Geometry: see drawing. Coordinates: mm, zero at the bounding-box minimum. Round coordinates to 2 decimals unless told otherwise and drop trailing zeros. Loops run counter-clockwise (first coordinate to the right, second up) from the corner with the lowest first, then second, coordinate; pieces in that order, holes last.
(1) Line query: line 1 (X direction, y = 1.55, z = 105); line 2 (Z direction, x = 5, y = 2.95); line 3 (Z direction, x = 5.5, y = 1.7). Output: solid intervals per line, ascending.
(2) Cut plane A-A, the plane z = 105. Output: boundary loops of the cut face in (x, y), and give its area (3 significant figures).
(3) First-contact query: pin 1 Ø8 at (x, z) = (13.5, 29) entering from -Y; pin 2 Ø1.9 at (x, z) = (5, 105) entering from +Y. Flat tips, straight axial feed; report the tip coordinate or a pass-through.
(4) Cut plane B-B, the plane x = 70. Output: boundary loops of the cut face in (y, z).
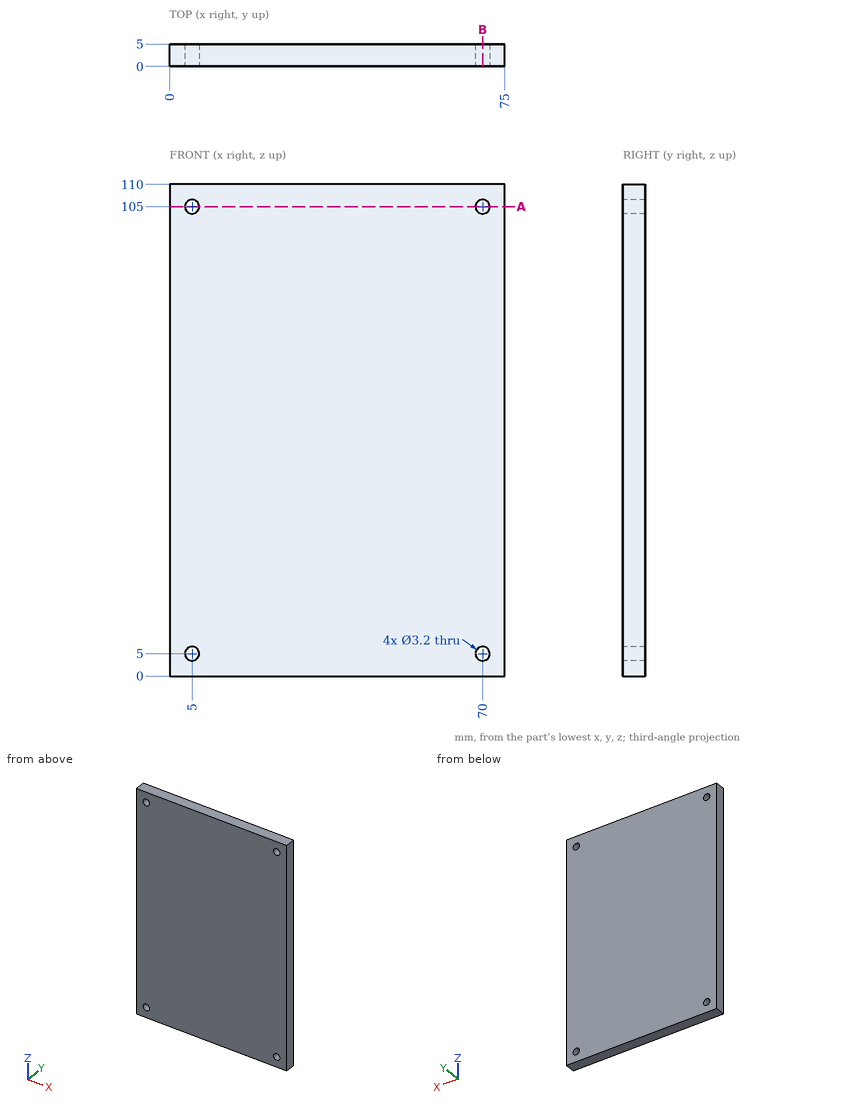
Reported:
1. line 1: x = 0 to 3.4, 6.6 to 68.4, 71.6 to 75
1. line 2: z = 0 to 3.4, 6.6 to 103.4, 106.6 to 110
1. line 3: z = 0 to 3.48, 6.52 to 103.48, 106.52 to 110
2. outline: (0, 0) - (3.4, 0) - (3.4, 5) - (0, 5) - close; (6.6, 0) - (68.4, 0) - (68.4, 5) - (6.6, 5) - close; (71.6, 0) - (75, 0) - (75, 5) - (71.6, 5) - close
2. area: 343 mm2
3. pin 1: stops at y = 0
3. pin 2: passes through
4. outline: (0, 0) - (5, 0) - (5, 3.4) - (0, 3.4) - close; (0, 6.6) - (5, 6.6) - (5, 103.4) - (0, 103.4) - close; (0, 106.6) - (5, 106.6) - (5, 110) - (0, 110) - close
